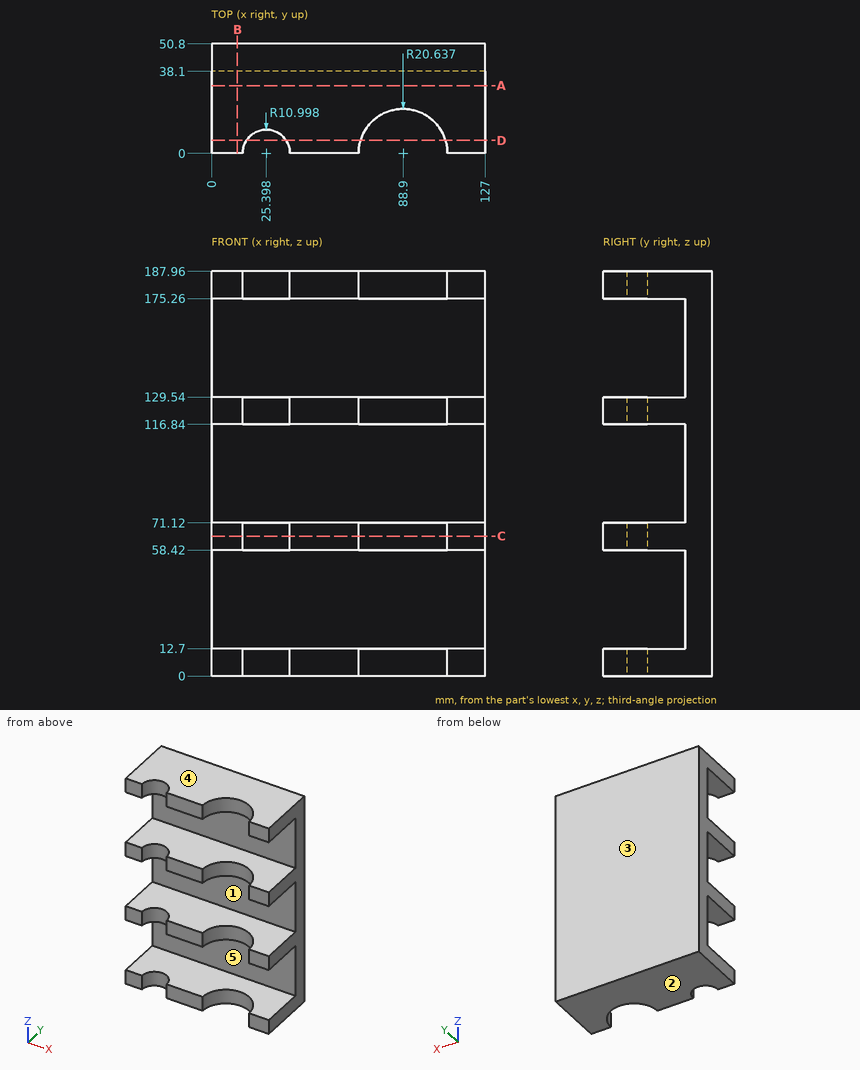
Design review of the part shown in the three views and the two pictorial views. Dimensions are in mm from the part's minimum x, y and z. A direction names the side the tool comes from. Give positions to 0.01 mm unless a question says otherwise; leave off trailing zeros. Write each loop counter-clockwise with the first axis right and the second up, starting at its lowest first coordinate (ties: lowest second). Pieces come first, ordered by that corner, then holes. Notation, with made-up numbers: (-20.75, -5.5) -> (-10.75, -5.5) arc R26 cw to (-10.75, 30.5) -> close; hole circle Ø1 at (0, -2.75). An arc over 180 degrees is marked (long way). Answer in a Markdown table with one row per item.
1) Add section C-C on z = 65. State the section outline as (x, y) points (1 decimal).
Worked answers:
| item | result |
|---|---|
| outline | (0, 0) -> (14.4, 0) arc R11 cw to (36.4, 0) -> (68.3, 0) arc R20.6 cw to (109.5, 0) -> (127, 0) -> (127, 50.8) -> (0, 50.8) -> close |
2) Add section D-D on y = 6. Count the separate pieces of the cut face and the enclosed holes in it, plus the area to 3 significant figures.
Worked answers:
| item | result |
|---|---|
| separate pieces | 12 |
| enclosed holes | 0 |
| area | 3,510 mm² |
3) Add section A-A on y = 31.5. State the section outline as (x, z) points.
Worked answers:
| item | result |
|---|---|
| outline | (0, 0) -> (127, 0) -> (127, 12.7) -> (0, 12.7) -> close; (0, 58.42) -> (127, 58.42) -> (127, 71.12) -> (0, 71.12) -> close; (0, 116.84) -> (127, 116.84) -> (127, 129.54) -> (0, 129.54) -> close; (0, 175.26) -> (127, 175.26) -> (127, 187.96) -> (0, 187.96) -> close |
4) Tool access review of the marked faces 4 and 5: name each direction out of +Z, -Z, +X, -X, +Y, -Y from which nothing blocks a thin tool from reaching the whole face with its end or side.
Worked answers:
| item | result |
|---|---|
| face 4 | +Z, +X, -X, +Y, -Y |
| face 5 | +X, -X, -Y |
5) For L1, parallel to Z at x = 17, y = 9; L2, parallel to X at y = 5, z = 120.5 (1 decimal); L3, parallel to Y at x = 39, z = 151, list the stretches that pass through material, from the lowest coordinate up. Write a range as [from, to].
Worked answers:
| item | result |
|---|---|
| L1 | [0, 12.7], [58.42, 71.12], [116.84, 129.54], [175.26, 187.96] |
| L2 | [0, 15.6], [35.2, 68.9], [108.9, 127] |
| L3 | [38.1, 50.8] |
6) Clearance check with flat-ended pins moving along their axes: P1, Ø13.5, axis at x = 62.5, z = 46, coming from the -Y side; P2, Ø1.5, axis at x = 84, z = 61, coming from the -Y side. State where each tip first meets the part, or that it passes through.
Worked answers:
| item | result |
|---|---|
| P1 | y = 38.1 |
| P2 | y = 19.85 |
7) Add section B-B on x = 12. State the section outline as (y, z) points.
Worked answers:
| item | result |
|---|---|
| outline | (0, 0) -> (50.8, 0) -> (50.8, 187.96) -> (0, 187.96) -> (0, 175.26) -> (38.1, 175.26) -> (38.1, 129.54) -> (0, 129.54) -> (0, 116.84) -> (38.1, 116.84) -> (38.1, 71.12) -> (0, 71.12) -> (0, 58.42) -> (38.1, 58.42) -> (38.1, 12.7) -> (0, 12.7) -> close |
8) Mouldability with a two-part tool opening along Z and no side actions: class the marked faces 1, 2 and 3 as +Z half, -Z half, draft (parallel to the pull), parting line (faces both ways), or undercut.
Worked answers:
| item | result |
|---|---|
| face 1 | undercut |
| face 2 | -Z half |
| face 3 | draft |
